The model under review builds one solid part; all positions refer to its coordinate system, in mm. A direction names the side the tool comes from. Coordinates: 2 decimals unless noted, no trailing zeros. Use one line per item in the form item = value. Start each with the question number.
(1) Wall thickness on line 1 along X through (y, z) = (-2.25, -19.05) (3 decimals); line 2 along X through (y, z) = (-2.25, -20) (3 decimals): over which ranges is each line inside the solid? List them lowest first.
(2) Mouldability with a two-part tool opening along Z and no side actions: class faces 3 (the flat face through (-2, 0, -31.75)), 4 (the conical face through (146.61, -8.66, 22.05)), 5 (the flat face through (-2, 9.525, 0)), 6 (the cylindrical face through (0.73, 1.15, -15.75)) as +Z half, -Z half, draft (parallel to the pull), parting line (faces both ways), or undercut.
(3) Insertion check: pin 1 Ø5.5 at (x, z) = (146.05, 22.225) entering from +Y; pin 2 Ø6 at (x, z) = (53.975, -19.05) entering from +Y. Each pin has a flat end and moves straight along its axis. Give the tip position at first contact, or say it passes through.
(4) For faces 1 (the cylindrical face through (149.425, 1.154, 22.076)), 2 (the flat face through (155.575, 0, 0)), list the 3-axis set-ups (+Z, -Z, +X, -X, +Y, -Y) from which the entire face can be reached by the end or side of a thin tool; tool diameter is ignored.
```python
from build123d import *

# Parameters (mm, degrees)
SKETCH1_W                   = 311.15
SKETCH1_H                   = 63.5
BOSS_EXTRUDE1_DEPTH         = 9.525
F_1_4_CLEARANCE_HOLE1_D     = 6.7564
F_1_4_CLEARANCE_HOLE1_DEPTH = 16.51
F_1_4_CLEARANCE_HOLE1_TIP   = 2.029827343


with BuildPart() as part:
    # Sketch1 → Boss-Extrude1 (new, symmetric)
    with BuildSketch(Plane(origin=(0, 0, 0), x_dir=(1, 0, 0), z_dir=(0, 1, 0))):
        Rectangle(SKETCH1_W, SKETCH1_H)
    extrude(amount=BOSS_EXTRUDE1_DEPTH, both=True)

    # 1/4 Clearance Hole1
    with Locations(Plane(origin=(0, 9.525, 0), x_dir=(1, 0, 0), z_dir=(0, 1, 0))):
        with Locations((-53.975, 19.05), (0, 19.05), (53.975, 19.05), (146.05, -22.225), (-146.05, -22.225)):
            Hole(F_1_4_CLEARANCE_HOLE1_D / 2, depth=F_1_4_CLEARANCE_HOLE1_DEPTH)
            with Locations((0, 0, -(F_1_4_CLEARANCE_HOLE1_DEPTH + F_1_4_CLEARANCE_HOLE1_TIP / 2))):  # 118° drill point
                Cone(0, F_1_4_CLEARANCE_HOLE1_D / 2, F_1_4_CLEARANCE_HOLE1_TIP, mode=Mode.SUBTRACT)


solid = part.part
```
Findings:
q1.line_1 = -155.575 to -57.353, -50.597 to -3.378, 3.378 to 50.597, 57.353 to 155.575
q1.line_2 = -155.575 to -57.217, -50.733 to -3.242, 3.242 to 50.733, 57.217 to 155.575
q2.face_3 = -Z half
q2.face_4 = undercut
q2.face_5 = draft
q2.face_6 = undercut
q3.pin_1 = -7.36
q3.pin_2 = -7.21
q4.face_1 = +Y
q4.face_2 = +Z, -Z, +X, +Y, -Y
